Autodesk Inventor part; units mm, degrees
ref_plane "Work Plane3" through (10.9593, -73.9067, -37.25) normal (-0.9081432, 0.4186597, 0) x (0, 0, 1)
ref_plane "Work Plane4" through (64.6996, 102.2233, -25) normal (-0.9187912, 0.3947439, 0) x (0, 0, 1)
ref_plane "Work Plane5" through (32.5419, 116.0393, -25) normal (-0.9187912, 0.3947439, 0) x (0, 0, 1)
sketch "Sketch1" plane through (0, 0, 0) normal (0, 1, 0) x (-1, 0, 0)
  line L0 (5.5, 37.25) -> (-5.5, 37.25)
  line L1 (-5.5, 37.25) -> (-5.5, -37.25)
  line L2 (-5.5, -37.25) -> (5.5, -37.25)
  line L3 (5.5, -37.25) -> (5.5, 37.25)
  line L4 (5.5, 37.25) -> (-5.5, -37.25) construction
  line L5 (-5.5, 37.25) -> (5.5, -37.25) construction
  circle A0 centre (0, 30) radius 1.5
  line L6 (5.5, 0) -> (-5.5, 0)
  circle A1 centre (0, -30) radius 1.5
  line L7 (-5.5, -25) -> (5.5, -25)
  line L8 (5.5, -25) -> (5.5, 25)
  line L9 (5.5, 25) -> (-5.5, 25)
  line L10 (-5.5, 25) -> (-5.5, -25)
  line L11 (-5.5, -25) -> (5.5, 25) construction
  line L12 (5.5, -25) -> (-5.5, 25) construction
  point P0 (0, 0)
  dimension "d0" = 11
  dimension "d1" = 74.5
  dimension "d2" = 3
  dimension "d3" = 7.25
  dimension "d28" = 50
extrude "Extrusion1" add sketch "Sketch1" along normal blind 10
sketch "Sketch2" plane through (5.5, 0, 37.25) normal (1, 0, 0) x (0, 0, -1)
  line L0 (0, 10) -> (74.5, 10)
  line L1 (0, 0) -> (74.5, 0)
  line L2 (0, 10) -> (74.5, 10)
  line L3 (74.5, 10) -> (74.5, 0)
  line L4 (74.5, 0) -> (0, 0)
  line L5 (0, 0) -> (0, 10)
  point P0 (37.25, 0)
extrude "Extrusion2" add sketch "Sketch2" along normal blind 10
sketch "Sketch3" plane through (0, 0, 0) normal (0, -1, 0) x (1, 0, 0)
  line L0 (-5.5, 37.25) -> (15.5, 37.25)
  line L1 (-5.5, -37.25) -> (15.5, -37.25)
  line L2 (15.5, 37.25) -> (4.8, 37.25)
  line L3 (4.8, 37.25) -> (4.8, -37.25)
  line L4 (4.8, -37.25) -> (15.5, -37.25)
  line L5 (15.5, -37.25) -> (15.5, 37.25)
  point P0 (0, 0)
  dimension "d9" = 10.7
extrude "Extrusion3" add sketch "Sketch3" along normal blind 76
ref_plane "Work Plane1" through (15.5, -76, -37.25) normal (-0.9081432, 0.4186597, 0) x (0, 0, 1)
ref_plane "Work Plane3" through (10.9593, -73.9067, -37.25) normal (-0.9081432, 0.4186597, 0) x (0, 0, 1)
sketch "Sketch4" plane through (10.9593, -73.9067, -37.25) normal (-0.9081432, 0.4186597, 0) x (0, 0, 1)
  circle A0 centre (37.25, 54.5) radius 2
  circle A1 centre (37.25, 54.5) radius 5.5
  circle A2 centre (27.25, 30.8) radius 2
  circle A3 centre (27.25, 30.8) radius 5.5
  line L0 (37.25, 62.5297) -> (37.25, 0)
  line L1 (0, 0) -> (74.5, 0)
  circle A4 centre (47.25, 30.8) radius 5.5
  circle A5 centre (47.25, 30.8) radius 2
  point P0 (37.25, 0)
  dimension "d13" = 4
  dimension "d14" = 11
  dimension "d15" = 4
  dimension "d16" = 11
  dimension "d19" = 10
  dimension "d20" = 23.7
  dimension "d23" = 54.5
extrude "Extrusion4" cut sketch "Sketch4" along normal blind 15 contours A0 L0 | A0 L0 A1 | L0 A0 | A0 L0 A1 | A2 | A3 | A4 | A5
extrude "Extrusion11" cut sketch "Sketch4" along normal blind 25.925 contours A0 L0 | A0 L0 A1 | L0 A0 | A0 L0 A1
extrude "Extrusion6" cut sketch "Sketch4" along normal through all contours A0 L0 | L0 A0 | A2 | A5
extrude "Extrusion7" add sketch "Sketch1" along normal blind 125 contours L3 L6 L1 L9 | L3 L7 L1 L6
sketch "Sketch5" plane through (5.5, 10, -25) normal (1, 0, 0) x (0, 0, -1)
  line L0 (0, 0) -> (0, 115)
  line L1 (0, 115) -> (0, 0)
  line L2 (0, 0) -> (-50, 0)
  line L3 (-50, 0) -> (-50, 115)
  line L4 (0, 115) -> (-50, 115)
  point P0 (-25, -10)
extrude "Extrusion8" add sketch "Sketch5" along normal blind 40
chamfer "Chamfer1" distance 40 angle 23.25 1 edges at (-5.5, 125, 0) measured on face at (-5.5, 48.3333, -8.3333)
chamfer "Chamfer2" distance 30 distance2 30 1 edges at (15.5, 10, 0)
sketch "Sketch8" plane through (11.6854, 125, -25) normal (-0.9187912, 0.3947439, 0) x (0, 0, 1)
  line L0 (0, 0) -> (0, 13.3481)
  line L1 (-12.25, -121.6327) -> (62.25, -121.6327)
  line L2 (0, 13.3481) -> (50, 13.3481)
  line L3 (50, 13.3481) -> (50, -121.6327)
  line L4 (50, -121.6327) -> (0, -121.6327)
  line L5 (0, -121.6327) -> (0, 13.3481)
  point P0 (25, -119.4616)
  point P1 (0, 0)
  dimension "d59" = 50
extrude "Extrusion12" cut sketch "Sketch8" against normal blind 22.7
ref_plane "Work Plane4" through (64.6996, 102.2233, -25) normal (-0.9187912, 0.3947439, 0) x (0, 0, 1)
ref_plane "Work Plane5" through (32.5419, 116.0393, -25) normal (-0.9187912, 0.3947439, 0) x (0, 0, 1)
ref_plane "Work Plane6" through (-5.5, 27.4944, -18.625) normal (0.3947439, 0.9187912, 0) x (0, 0, -1)
sketch "Sketch11" plane through (15.5, 10, -25) normal (0, 0, -1) x (-1, 0, 0)
  line L0 (21, 17.4944) -> (-6.8294, 82.2691)
  line L1 (21, 17.4944) -> (11, 17.4944)
  line L2 (11, 17.4944) -> (11, 13.4944)
  line L3 (11, 13.4944) -> (21, 13.4944)
  line L4 (21, 13.4944) -> (21, 17.4944)
  point P0 (15.5, -10)
  dimension "d76" = 10
  dimension "d77" = 4
extrude "Extrusion15" cut sketch "Sketch11" against normal blind 70.5
fillet "Fillet1" radius 5 2 edges at (15.5, -33, 37.25) (15.5, -33, -37.25)
sketch "Sketch12" plane through (32.5419, 116.0393, -25) normal (-0.9187912, 0.3947439, 0) x (0, 0, 1)
  line L0 (6, -0.2473) -> (44, -0.2473)
  line L1 (44, -0.2473) -> (44, -96.0989)
  line L2 (6, -96.0989) -> (6, -0.2473)
  line L3 (0, -96.3711) -> (0, 9.7527)
  line L4 (50, 9.7527) -> (50, -96.3711)
  line L5 (0, 9.7527) -> (50, 9.7527)
  line L6 (44, -96.0989) -> (44, -96.8375)
  line L7 (44, -96.8375) -> (6, -96.8375)
  line L8 (6, -96.8375) -> (6, -96.0989)
  point P0 (25, -119.4616)
  dimension "d81" = 6
  dimension "d82" = 6
  dimension "d83" = 10
extrude "Extrusion16" cut sketch "Sketch12" against normal blind 9
sketch "Sketch14" plane through (4.5, 23.4944, -25) normal (-1, 0, 0) x (0, 0, 1)
  line L0 (6, 4) -> (6, 92.3177)
  line L1 (6, 4) -> (44, 4)
  line L2 (44, 4) -> (44, 0)
  line L3 (44, 0) -> (6, 0)
  line L4 (6, 0) -> (6, 4)
  point P0 (25, -23.4944)
  point P1 (6, 19)
extrude "Extrusion18" cut sketch "Sketch14" against normal blind 7
sketch "Sketch15" plane through (15.5, 10, -25) normal (0, 0, -1) x (-1, 0, 0)
  line L0 (-30, 115) -> (-39.6875, 115)
  line L1 (-39.6875, 115) -> (-39.6875, 9.6875)
  line L2 (-30, 0) -> (-39.6875, 9.6875)
  line L3 (0, -30) -> (-30, 0)
  line L4 (21, 13.4944) -> (11, 13.4944)
  line L5 (11, 13.4944) -> (11, 17.4944)
  line L6 (11, 17.4944) -> (21, 17.4944)
  line L7 (21, 17.4944) -> (-20.8917, 115) construction
  line L8 (-20.8917, 115) -> (-30, 115)
  line L9 (-30, 0) -> (-30, 115)
  line L10 (0, -30) -> (-30, 0)
  line L11 (0, 0) -> (0, -30)
  line L12 (21, 0) -> (0, 0)
  line L13 (21, 0) -> (21, 13.4944)
  point P0 (15.5, -10)
  dimension "d91" = 135
extrude "Extrusion19" add sketch "Sketch15" against normal blind 50
sketch "Sketch16" plane through (40.811, 112.4866, -25) normal (-0.9187912, 0.3947439, 0) x (0, 0, 1)
  line L0 (6, -96.3711) -> (6, -0.2473)
  line L1 (44, -93.3357) -> (6, -93.3357)
  line L2 (6, -0.2473) -> (44, -0.2473)
  line L3 (44, -0.2473) -> (44, -93.3357)
  line L4 (44, -93.3357) -> (6, -93.3357)
  line L5 (6, -93.3357) -> (6, -0.2473)
  point P0 (25, -119.4616)
extrude "Extrusion20" cut sketch "Sketch16" against normal blind 9
sketch "Sketch18" plane through (49.0802, 108.9339, -25) normal (-0.9187912, 0.3947439, 0) x (0, 0, 1)
  line L0 (6, -0.2473) -> (44, -0.2473) construction
  line L1 (25, -0.2473) -> (25, -12.2473) construction
  line L2 (6, -93.3357) -> (6, -0.2473) construction
  line L3 (44, -0.2473) -> (44, -93.3357) construction
  circle A0 centre (25, -12.2473) radius 3.5
  circle A1 centre (25, -27.2473) radius 3.5
  point P0 (25, -119.4616)
  dimension "d99" = 12
  dimension "d100" = 19
  dimension "d103" = 7
  dimension "d104" = 7
  dimension "d105" = 15
extrude "Extrusion22" cut sketch "Sketch18" against normal through all
ref_plane "Work Plane8" through (72.0499, 99.0653, -25) normal (-0.9187912, 0.3947439, 0) x (0, 0, 1)
sketch "Sketch19" plane through (72.0499, 99.0653, -25) normal (-0.9187912, 0.3947439, 0) x (0, 0, 1)
  circle A0 centre (25, -12.2473) radius 3.5
  circle A1 centre (25, -12.2473) radius 6
  circle A2 centre (25, -27.2473) radius 3.5
  circle A3 centre (25, -27.2473) radius 6
  point P0 (25, -119.4616)
  dimension "d109" = 12
  dimension "d110" = 12
extrude "Extrusion23" cut sketch "Sketch19" along normal blind 15 contours A3
extrude "Extrusion24" cut sketch "Sketch19" along normal blind 20 contours A1
sketch "Sketch20" plane through (-5.5, 10, 25) normal (0, 0, 1) x (1, 0, 0)
  line L0 (21, -30) -> (60.6875, 9.6875)
  line L1 (57.35, 6.35) -> (57.35, 115)
  line L2 (41.8917, 115) -> (60.6875, 115)
  line L3 (57.35, 115) -> (87.3125, 115)
  line L4 (87.3125, 115) -> (90.4875, 6.35)
  line L5 (90.4875, 6.35) -> (57.35, 6.35)
  point P0 (5.5, -10)
extrude "Extrusion25" cut sketch "Sketch20" against normal through all
properties part number "Camera Bracket"
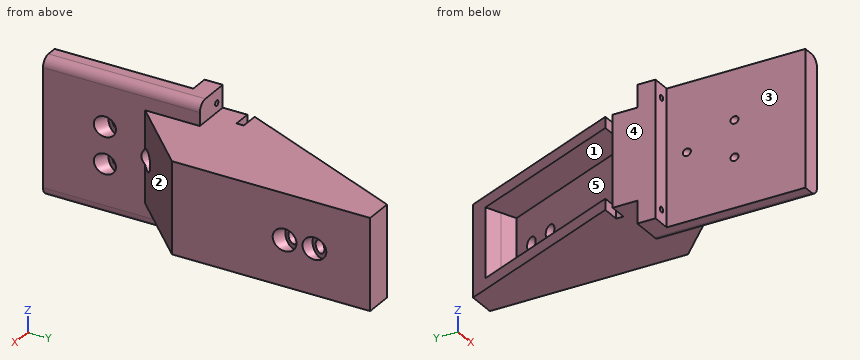
Input: part model. Units: mm. Frame: model coordinates. Face numbers are marked on the shaded views. A direction names the side the tool comes from. Give positions to 0.01 mm unless a question says otherwise; leave off trailing zeros. Loops run counter-clockwise (first coordinate to the right, second up) from the corner with the lowest first, then second, coordinate; pieces in that order, holes last. Notation, with made-up numbers: M -27,45.5 L 29,45.5 A28 cw 29,78.5 Z; hole C -32.75,-31.75 d1. An arc over 180 degrees is marked long. Use one line per item in the form item = value.
1. First-contact query: pin 1 (5 mm diameter, centred on x = 2, z = -8.5, fed in from -Y); pin 2 (5 mm diameter, centred on y = 74, z = -14.5, fed in from -X); pin 3 (3.5 mm diameter, centred on x = 8, z = 33, fed in from +Y). Flat tips, straight axial feed; report the tip coordinate or a pass-through.
Numbers:
pin_1 = 0
pin_2 = 33
pin_3 = 10
2. Reachability of the marked faces 1, 2 and 3 from +Z, -Z, +X, -X, +Y, -Y: full face, straight path, thin tool, end or side. Return the list, or none.
Numbers:
face_1 = -X
face_2 = +Z, -Z, +X, -Y
face_3 = +Z, -Z, -X, -Y
3. Section query A-A, the plane y = 52.5. Return the cut outline in (x, z), and give its area (3 significant figures).
Numbers:
outline = M 5.25,-25 L 51.85,-25 L 51.85,25 L 5.25,25 L 5.25,19 L 24.84,19 L 24.84,-19 L 5.25,-19 Z
area = 1,590 mm²
4. Pull-direction query (Z, two-part tool) for the marked faces 4 and 5; classes: released by +Z, released by -Z, zero draft, split by the parting line, or undercut.
Numbers:
face_4 = zero draft
face_5 = undercut
5. Line query: L1, parallel to Z at x = 0, y = 5.25; L2, parallel to Y at x = 44.5, z = 2; L3, parallel to Z at x = 1, y = 3. Output: solid intervals per line, ascending.
Numbers:
L1 = -37.25 to -31.5, -28.5 to 28.5, 31.5 to 37.25
L2 = 9 to 78.12, 84.37 to 94.45, 110.63 to 125
L3 = -37.25 to -31.12, -28.88 to 28.88, 31.12 to 37.25
